from build123d import *

# Parameters (mm, degrees)
F0_R        = 0.85
F1_DEPTH    = 1
F2_T1_DEPTH = 1
F3_R        = 5


# Not quite as in the source:
# - a fillet or chamfer that OpenCascade refuses, or shapes differently, is made with other operations: its cross-section is extruded or revolved along the edge and cut away or added


with BuildPart() as f1:
    # F0 (on Front) → F1 (new body)
    with BuildSketch(Plane.XZ):
        with BuildLine():
            ThreePointArc((-0.85, -6.6458633751), (0, 6.7), (0.85, -6.6458633751))
            Line((0.85, -6.6458633751), (0.85, -10.1645216316))
            ThreePointArc((0.85, -10.1645216316), (3.1164454592, -9.7122483339), (5.2228952278, -8.7613563698))
            Line((5.2228952278, -8.7613563698), (4.5, -7.2111025509))
            ThreePointArc((4.5, -7.2111025509), (0, 8.8), (-4.5, -7.2111025509))
            Line((-4.5, -7.2111025509), (-5.2228952278, -8.7613563698))
            ThreePointArc((-5.2228952278, -8.7613563698), (-3.1164454592, -9.7122483339), (-0.85, -10.1645216316))
            Line((-0.85, -10.1645216316), (-0.85, -6.6458633751))
        make_face()
        with Locations((-2.5559992958, -8.1065940814)):
            Circle(F0_R, mode=Mode.SUBTRACT)
        with Locations((2.5559992958, -8.1065940814)):
            Circle(F0_R, mode=Mode.SUBTRACT)
    extrude(amount=F1_DEPTH)

    # F2: fillet of radius 10 on 2 edges, made by hand

    # F2_s2 → F2_t1 (join)
    with BuildSketch(Plane.XZ):
        with BuildLine():
            ThreePointArc((-6.9462853719, -4.9724032485), (-5.8852649135, -6.7762174559), (-5.2228952278, -8.7613563698))
            Line((-5.2228952278, -8.7613563698), (-4.5, -7.2111025509))
            ThreePointArc((-4.5, -7.2111025509), (-5.8315783323, -6.210243371), (-6.9462853719, -4.9724032485))
        make_face()
        with BuildLine():
            ThreePointArc((5.2228952278, -8.7613563698), (5.8852649135, -6.7762174559), (6.9462853719, -4.9724032485))
            ThreePointArc((6.9462853719, -4.9724032485), (5.8315783323, -6.210243371), (4.5, -7.2111025509))
            Line((4.5, -7.2111025509), (5.2228952278, -8.7613563698))
        make_face()
    extrude(amount=F2_T1_DEPTH)

    # F3
    f3_edges = [f1.edges().sort_by_distance(p)[0] for p in [
        (-5.222895, -0.5, -8.761356),
        (5.222895, -0.5, -8.761356),
    ]]
    fillet(f3_edges, radius=F3_R)


solid = f1.part
Work out the finished part from the listing and answer in its coordinate system (mm). A direction names the side the tool comes from. Give positions to 0.01 mm unless a question says otherwise; leave off trailing zeros. Order: outer loops, then holes, each group sorted by start corner. A loop starts at its lowest first (then second) coordinate and runs counter-clockwise, first axis right, second up. Notation, with made-up numbers: (74.25, -8.75) -> (124.25, -8.75) arc R27 cw to (124.25, 27.25) -> close; hole circle Ø2 at (7, 18.25). An arc over 180 degrees is marked (long way). Answer as a JSON object with one key per item and string values. Group by question number.
1. The mould has two halves that part along Z. Classify faces 3 (the cylindrical face through (-1.593, -0.493, -10.075)), 4 (the cylindrical face through (0.267, -0.493, 8.796)), 5 (the cylindrical face through (-2.667, -0.493, -7.264)): released by +Z, released by -Z, zero draft, split by the parting line, or undercut.
2. A tool of negligible diameter and unlimited length cuts with its end or side. For faces 1 (the flat face through (-4, 0, -6)), 2 (the flat face through (0.85, -0.5, -8.4)), from which of +Z, -Z, +X, -X, +Y, -Y can it reach the whole face along a straight path? Write none if from no direction.
3. Section C-C on x = -3 is taken. Count the separate pieces of the cut face and the enclosed holes in it, plus the area to 3 significant figures.
4. Section A-A on z = 5.25 is taken. Determine the outline of the cut face in (x, y).
5. Flat-ended cylindrical pins translate along their axes: pin 1 Ø4 at (x, z) = (-2, 3) entering from +Y; pin 2 Ø0.5 at (y, z) = (-0.5, -8.5) entering from -X; pin 3 Ø0.5 at (y, z) = (-0.5, -9) entering from +X. Find the tip coordinate at first contact, or state that the pin passes through.
6. Section B-B on z = -6 is taken. Determine the outline of the cut face in (x, y).
7. Consider line 1 along X through (y, z) = (-0.6, 0); line 2 along X through (y, z) = (-0.3, -8); line 3 along Z through (x, y) = (-2.75, -0.85). Determine where each line is inside the solid, lowest interval first. Write a range as [from, to].
Result sheet:
{
 "1": {"face 3": "released by -Z", "face 4": "split by the parting line", "face 5": "undercut"},
 "2": {"face 1": "+Z, -Z, +X, -X, +Y", "face 2": "-Z, +Y, -Y"},
 "3": {"separate pieces": "3", "enclosed holes": "0", "area": "4.55 mm^2"},
 "4": {"outline": "(-6.98, -1) -> (-4.16, -1) -> (-4.16, 0) -> (-6.98, 0) -> close; (4.16, -1) -> (6.98, -1) -> (6.98, 0) -> (4.16, 0) -> close"},
 "5": {"pin 1": "passes through", "pin 2": "stops at x = -5.03", "pin 3": "stops at x = 4.56"},
 "6": {"outline": "(-6.28, -1) -> (-2.98, -1) -> (-2.98, 0) -> (-6.28, 0) -> close; (2.98, -1) -> (6.28, -1) -> (6.28, 0) -> (2.98, 0) -> close"},
 "7": {"line 1": "x = [-8.64, -6.7], [6.7, 8.64]", "line 2": "x = [-5.22, -3.4], [-1.71, -0.85], [0.85, 1.71], [3.4, 5.22]", "line 3": "z = [-9.81, -8.93], [-7.28, -6.11], [6.11, 8.35]"}
}
